```python
from build123d import *

# Parameters (mm, degrees)
SKETCH1_W           = 7
SKETCH1_H           = 7
BOSS_EXTRUDE1_DEPTH = 3
CUT_EXTRUDE1_DEPTH  = 7
CUT_EXTRUDE2_DEPTH  = 11
SKETCH4_R           = 1.8
CUT_EXTRUDE3_DEPTH  = 0.8
CUT_EXTRUDE4_DEPTH  = 0.4


with BuildPart() as part:
    # Sketch1 → Boss-Extrude1 (new body)
    with BuildSketch(Plane(origin=(0, 0, 0), x_dir=(1, 0, 0), z_dir=(0, 1, 0))):
        with Locations((3.5, 3.5)):
            Rectangle(SKETCH1_W, SKETCH1_H)
    extrude(amount=BOSS_EXTRUDE1_DEPTH)

    # Sketch2 → Cut-Extrude1 (cut)
    with BuildSketch(Plane.XY):
        Polygon((0, 0), (0.7, 3), (0, 3), align=None)
        Polygon((7, 0), (6.3, 3), (7, 3), align=None)
    extrude(amount=-CUT_EXTRUDE1_DEPTH, mode=Mode.SUBTRACT)

    # Sketch3 → Cut-Extrude2 (cut)
    with BuildSketch(Plane(origin=(0, 0, 0), x_dir=(0, 0, -1), z_dir=(1, 0, 0))):
        Polygon((0, 0), (0.7, 3), (0, 3), align=None)
        Polygon((7, 3), (6.3, 3), (7, 0), align=None)
    extrude(amount=CUT_EXTRUDE2_DEPTH, mode=Mode.SUBTRACT)

    # Sketch4 → Cut-Extrude3 (cut)
    with BuildSketch(Plane.XZ):
        with Locations(Location((3.5, -3.5, 0), (0, 0, 270))):
            Circle(SKETCH4_R)
    extrude(amount=-CUT_EXTRUDE3_DEPTH, mode=Mode.SUBTRACT)

    # Sketch5 → Cut-Extrude4 (cut)
    with BuildSketch(Plane(origin=(0, 3, 0), x_dir=(1, 0, 0), z_dir=(0, 1, 0))):
        Polygon((3.18174557, 1.759282352), (1.887474737, 5.259282352), (2.598412237, 5.259282352), (3.525295249, 2.656718249), (4.448672653, 5.259282352), (5.163115762, 5.259282352), (3.873752781, 1.759282352), align=None)
    extrude(amount=-CUT_EXTRUDE4_DEPTH, mode=Mode.SUBTRACT)


solid = part.part
```
Input: part model. Units: mm. Frame: model coordinates. A direction names the side the tool comes from. Round coordinates to 2 decimals unless told otherwise and drop trailing zeros. Loops run counter-clockwise (first coordinate to the right, second up) from the corner with the lowest first, then second, coordinate; pieces in that order, holes last.
1) Set-up query: faces 4 (the flat face through (3.055, 2.803, -3.976)), 5 (the flat face through (6.655, 1.479, -3.451)), 6 (the flat face through (4, 0.8, -3)). Return all of +Z, -Z, +X, -X, +Y, -Y with unobstructed straight access to the full face (end or side cutting, diameter ignored); none if empty.
Ans:
face 4: +Y
face 5: +Z, -Z, +X, +Y
face 6: -Y
2) Material intervals for line 1 (Y direction, x = 4.5, z = -4); line 2 (X direction, y = 0.4, z = -3.5); line 3 (Z direction, x = 4, y = 0.45) (3 decimals), sorted ascending.
Ans:
line 1: y = 0.8 to 2.6
line 2: x = 0.09 to 1.7, 5.3 to 6.91
line 3: z = -6.895 to -5.229, -1.771 to -0.105
3) Section query A-A on x = 5.75. Return the cut outline in (y, z), plus the area to 3 significant figures.
Ans:
outline: (0, -7) - (3, -6.3) - (3, -0.7) - (0, 0) - close
area: 18.9 mm2
4) Pull-direction query (Z, two-part tool) for faces 1 (the flat face through (2.544, 2.803, -3.485)), 2 (the flat face through (2, 0, -5)), 3 (the flat face through (3.451, 1.521, -6.645)); classes: released by +Z, released by -Z, zero draft, split by the parting line, or undercut.
Ans:
face 1: undercut
face 2: zero draft
face 3: released by -Z
5) Pin query (flat end, axial travel): pin 1 (1 mm diameter, centred on y = 2, z = -2.5, fed in from +X). Return the tip coordinate at first contact, or that it passes through.
Ans:
pin 1: stops at x = 6.65
6) Section query C-C on z = -4.25. Return the cut outline in (x, y), plus the area to 3 significant figures.
Ans:
outline: (0, 0) - (1.86, 0) - (1.86, 0.8) - (5.14, 0.8) - (5.14, 0) - (7, 0) - (6.3, 3) - (4.79, 3) - (4.79, 2.6) - (4.09, 2.6) - (4.09, 3) - (2.96, 3) - (2.96, 2.6) - (2.26, 2.6) - (2.26, 3) - (0.7, 3) - close
area: 15.7 mm2
7) Section query D-D on y = 1.05. Return the cut outline in (x, z) (3 decimals), plus the area to 3 significant figures.
Ans:
outline: (0.245, -6.755) - (6.755, -6.755) - (6.755, -0.245) - (0.245, -0.245) - close
area: 42.4 mm2
8) Section query B-B on y = 0.2. Return the cut outline in (x, z), plus the area to 3 significant figures.
Ans:
outline: (0.05, -6.95) - (6.95, -6.95) - (6.95, -0.05) - (0.05, -0.05) - close; hole circle Ø3.6 at (3.5, -3.5)
area: 37.5 mm2
